Build history of the part. All positions in model axes, mm. A direction names the side the tool comes from. Give positions to 0.01 mm unless a question says otherwise; leave off trailing zeros. Write each loop counter-clockwise with the first axis right and the second up, starting at its lowest first coordinate (ties: lowest second). Pieces come first, ordered by that corner, then holes. Notation, with made-up numbers: M 30,22 L 65,22 A18 cw 65,53 Z; hole C 77.5,-32 d8. An arc over 180 degrees is marked long. Return JSON: item names as keys, results as strings. Group by question number.
Q1. Band-saw the part on D-D, the plane z = -24. Give the cut face in (x, y), then the cut area to 3 significant figures.
Q2. Band-saw the part on B-B, the plane y = 7.5. Count the separate pieces of the cut face and the enclosed holes in it, then the cut area to 3 significant figures.
Q3. Flat gauge pin, fed straight in: pin 1 Ø7.5 at (x, z) = (-17.5, 18.5) entering from -Y. Where does the tip first touch, or does it go through?
Q4. Pull direction X, two halves, no side cores. Call faces 3 (the flat face through (14, 3, -14)), 4 (the cylindrical face through (-29.65, 4.56, -29.49)), 5 (the flat face through (21.303, 2.958, 13.949)), 6 (the flat face through (0, 4, -32.5)): +X half, -X half, draft (parallel to the pull), parting line (faces both ways), or undercut.
Q5. Band-saw the part on C-C, the plane z = 0. Give the cut face in (x, y), then the cut area to 3 significant figures.
Q6. Tool access for faces 1 (the cylindrical face through (-20.217, 7.521, -15.731)), 2 (the flat face through (-13.949, 2.958, 21.303)): list every direction of +Z, -Z, +X, -X, +Y, -Y with a clear straight run to the whole face (end or side of a thin tool).
Q7. Band-saw the part on A-A, the plane x = 0. Give the cut face in (y, z).
Q8. Wall check: probe 1 along Z at (x, y) = (0, 2.75); probe 2 along Z at (x, y) = (15.5, 5.25). Give the ranges that are in metal, low to high.
from build123d import *

# Parameters (mm, degrees)
SKETCH_1_W          = 65
SKETCH_1_H          = 65
EXTRUDE_1_DEPTH     = 9
SKETCH_2_R          = 3.2
CUT_EXTRUDE_1_DEPTH = 9
CUT_EXTRUDE_2_DEPTH = 6
FILLET_1_R          = 10


with BuildPart() as part:
    # 스케치1 → 보스-돌출1 (new body)
    with BuildSketch(Plane(origin=(0, 0, 0), x_dir=(1, 0, 0), z_dir=(0, 1, 0))):
        Rectangle(SKETCH_1_W, SKETCH_1_H)
    extrude(amount=EXTRUDE_1_DEPTH)

    # 스케치2 → 컷-돌출1 (cut)
    with BuildSketch(Plane(origin=(0, 9, 0), x_dir=(1, 0, 0), z_dir=(0, 1, 0))):
        with Locations((-17.67766953, 17.67766953)):
            Circle(SKETCH_2_R)
        with Locations((17.67766953, -17.67766953)):
            Circle(SKETCH_2_R)
        with Locations((-17.67766953, -17.67766953)):
            Circle(SKETCH_2_R)
        with Locations((17.67766953, 17.67766953)):
            Circle(SKETCH_2_R)
        with Locations((0, 25)):
            Circle(SKETCH_2_R)
        with Locations((25, 0)):
            Circle(SKETCH_2_R)
        with Locations((0, -25)):
            Circle(SKETCH_2_R)
        with Locations((-25, 0)):
            Circle(SKETCH_2_R)
    extrude(amount=-CUT_EXTRUDE_1_DEPTH, mode=Mode.SUBTRACT)

    # 스케치3 → 컷-돌출2 (cut)
    with BuildSketch(Plane.XZ):
        Polygon((-25.031580054, 17.67766953), (-17.67766953, 10.323759005), (-10.323759005, 17.67766953), (-17.67766953, 25.031580054), align=None)
        Polygon((10.323759005, 17.67766953), (17.67766953, 10.323759005), (25.031580054, 17.67766953), (17.67766953, 25.031580054), align=None)
        Polygon((10.323759005, -17.67766953), (17.67766953, -25.031580054), (25.031580054, -17.67766953), (17.67766953, -10.323759005), align=None)
        Polygon((-25.031580054, -17.67766953), (-17.67766953, -25.031580054), (-10.323759005, -17.67766953), (-17.67766953, -10.323759005), align=None)
    extrude(amount=-CUT_EXTRUDE_2_DEPTH, mode=Mode.SUBTRACT)

    # 필렛1
    fillet_1_edges = [part.edges().sort_by_distance(p)[0] for p in [
        (-32.5, 4.5, -32.5),
        (32.5, 4.5, -32.5),
        (32.5, 4.5, 32.5),
        (-32.5, 4.5, 32.5),
    ]]
    fillet(fillet_1_edges, radius=FILLET_1_R)


solid = part.part
From the geometry:
{
 "1": {"outline": "M -32.39,0 L -18.71,0 L -18.71,6 L -16.65,6 L -16.65,0 L -3.04,0 L -3.04,9 L -32.39,9 Z; M 3.04,0 L 16.65,0 L 16.65,6 L 18.71,6 L 18.71,0 L 32.39,0 L 32.39,9 L 3.04,9 Z", "area": "503 mm^2"},
 "2": {"separate pieces": "1", "enclosed holes": "8", "area": "3,880 mm^2"},
 "3": {"pin 1": "stops at y = 6"},
 "4": {"face 3": "undercut", "face 4": "-X half", "face 5": "undercut", "face 6": "draft"},
 "5": {"outline": "M -32.5,0 L -28.2,0 L -28.2,9 L -32.5,9 Z; M -21.8,0 L 21.8,0 L 21.8,9 L -21.8,9 Z; M 28.2,0 L 32.5,0 L 32.5,9 L 28.2,9 Z", "area": "470 mm^2"},
 "6": {"face 1": "+Y, -Y", "face 2": "-Y"},
 "7": {"outline": "M 0,-32.5 L 9,-32.5 L 9,-28.2 L 0,-28.2 Z; M 0,-21.8 L 9,-21.8 L 9,21.8 L 0,21.8 Z; M 0,28.2 L 9,28.2 L 9,32.5 L 0,32.5 Z"},
 "8": {"probe 1": "z = -32.5 to -28.2, -21.8 to 21.8, 28.2 to 32.5", "probe 2": "z = -32.5 to -22.85, -12.5 to 12.5, 22.85 to 32.5"}
}
